Here's how the part is built. I have some questions about the finished solid (model axes, mm). A direction names the side the tool comes from. Round coordinates to 2 decimals unless told otherwise and drop trailing zeros. Loops run counter-clockwise (first coordinate to the right, second up) from the corner with the lowest first, then second, coordinate; pieces in that order, holes last. Notation, with made-up numbers: M 78.5,4.25 L 134.5,4.25 A32 ccw 134.5,39.25 Z; hole C 81.5,1.5 d6. An arc over 180 degrees is marked long. Put each result on its own line as item: value. Start each with the question number.
```python
from build123d import *

# Parameters (mm, degrees)
BOX019_W          = 3
BOX019_H          = 3
BOX019_DEPTH      = 10
CYLINDER022_R     = 3
CYLINDER022_DEPTH = 10
BOX020_W          = 87
BOX020_H          = 45
BOX020_DEPTH      = 12


with BuildPart() as cube019:
    # Box019 → Box019 (new body)
    with BuildSketch(Plane(origin=(-1.5, 2, 0), x_dir=(1, 0, 0), z_dir=(0, 0, 1))):
        with Locations((1.5, 1.5)):
            Rectangle(BOX019_W, BOX019_H)
    extrude(amount=BOX019_DEPTH)


with BuildPart() as fusion010:
    # Cylinder022 → Cylinder022 (new body)
    with BuildSketch(Plane.XY):
        Circle(CYLINDER022_R)
    extrude(amount=CYLINDER022_DEPTH)

    # Fusion010: union Cube019
    add(cube019.part)


with BuildPart() as kegel:
    # Cone → Cone (revolve)
    with BuildSketch(Plane.XZ):
        Polygon((0, 0), (7.5, 0), (10, 10), (0, 10), align=None)
    revolve(axis=Axis((0, 0, 0), (0, 0, 1)))


with BuildPart() as cut006:
    # Cut006 base: copy of Kegel
    add(kegel.part)

    # Cut006: cut Fusion010
    add(fusion010.part, mode=Mode.SUBTRACT)


with BuildPart() as cut006_1:
    # Cut006 placement: moved
    add(cut006.part.moved(Location((0, -21, 0))))


with BuildPart() as cut007:
    # Cut007 base: copy of Kegel
    add(kegel.part)

    # Cut007: cut Fusion010
    add(fusion010.part, mode=Mode.SUBTRACT)


with BuildPart() as cut007_1:
    # Cut007 placement: moved
    add(cut007.part.moved(Location((-42, -21, 0))))


with BuildPart() as cut008:
    # Cut008 base: copy of Kegel
    add(kegel.part)

    # Cut008: cut Fusion010
    add(fusion010.part, mode=Mode.SUBTRACT)


with BuildPart() as cut008_1:
    # Cut008 placement: moved
    add(cut008.part.moved(Location((21, 0, 0))))


with BuildPart() as cut009:
    # Cut009 base: copy of Kegel
    add(kegel.part)

    # Cut009: cut Fusion010
    add(fusion010.part, mode=Mode.SUBTRACT)


with BuildPart() as cut009_1:
    # Cut009 placement: moved
    add(cut009.part.moved(Location((-42, 0, 0))))


with BuildPart() as cut010:
    # Cut010 base: copy of Kegel
    add(kegel.part)

    # Cut010: cut Fusion010
    add(fusion010.part, mode=Mode.SUBTRACT)


with BuildPart() as cut011:
    # Cut011 base: copy of Kegel
    add(kegel.part)

    # Cut011: cut Fusion010
    add(fusion010.part, mode=Mode.SUBTRACT)


with BuildPart() as cut011_1:
    # Cut011 placement: moved
    add(cut011.part.moved(Location((-21, -21, 0))))


with BuildPart() as cut012:
    # Cut012 base: copy of Kegel
    add(kegel.part)

    # Cut012: cut Fusion010
    add(fusion010.part, mode=Mode.SUBTRACT)


with BuildPart() as cut012_1:
    # Cut012 placement: moved
    add(cut012.part.moved(Location((-21, 0, 0))))


with BuildPart() as fusion011:
    # Cut005 base: copy of Kegel
    add(kegel.part)

    # Cut005: cut Fusion010
    add(fusion010.part, mode=Mode.SUBTRACT)


with BuildPart() as fusion011_1:
    # Cut005 placement: moved
    add(fusion011.part.moved(Location((21, -21, 0))))

    # Fusion011: union Cut006, Cut007, Cut008, Cut009, Cut010, Cut011, Cut012
    add(cut006_1.part)
    add(cut007_1.part)
    add(cut008_1.part)
    add(cut009_1.part)
    add(cut010.part)
    add(cut011_1.part)
    add(cut012_1.part)


with BuildPart() as obj1:
    # Box020 → Box020 (new body)
    with BuildSketch(Plane(origin=(-54, -33, -2), x_dir=(1, 0, 0), z_dir=(0, 0, 1))):
        with Locations((43.5, 22.5)):
            Rectangle(BOX020_W, BOX020_H)
    extrude(amount=BOX020_DEPTH)

    # Cut013: cut Fusion011
    add(fusion011_1.part, mode=Mode.SUBTRACT)


solid = obj1.part
```
1) If we mould it in two halves opening along X, with no side actions, what happens to faces 3 (the face through (-42, -20, 10)), 4 (the face through (-48.5, -26, 2.8)), 5 (the face through (-22.5, 4, 5)), 6 (the face through (-54, -11, 4))? For each: pulls with the +X half, pulls with the -X half, needs draft (parallel to the pull), parting line crosses it, or undercut.
2) On a 3-axis mill with a long thin cutter (end or side, diameter ignored), from which of +Z, -Z, +X, -X, +Y, -Y can I reach the whole of each face in a straight line? I mean faces 1 (the face through (21, 1, 10)), 2 (the face through (0, 5, 5)). Say none if no direction works.
3) Suppose I cut it at A-A (z = 1). State how many separate pieces and enclosed holes the cut face has, plus the area to 3 significant figures.
4) Suppose I cut it at B-B (x = 21). Write out the boundary of the cut face in (y, z).
5) If I drill on probe 1 along Y at (x, z) = (-44, 9); probe 2 along Y at (x, z) = (2, 1); probe 3 along X at (y, z) = (-14.5, 8.25), over which ranges is the centre line in solid material (lowest first)? Write a range as from..to.
Results are:
1. face 3: needs draft
1. face 4: undercut
1. face 5: undercut
1. face 6: pulls with the -X half
2. face 1: +Z, +X, -X, +Y, -Y
2. face 2: +Z
3. separate pieces: 9
3. enclosed holes: 8
3. area: 2,680 mm²
4. outline: M -33,-2 L 12,-2 L 12,10 L 10,10 L 7.5,0 L 5,0 L 5,10 L -3,10 L -3,0 L -7.5,0 L -10,10 L -11,10 L -13.5,0 L -16,0 L -16,10 L -24,10 L -24,0 L -28.5,0 L -31,10 L -33,10 Z
5. probe 1: -33..-30.54, -23.24..-18.76, -11.46..-9.54, -2.24..2.24, 9.54..12
5. probe 2: -33..-28.49, -23.24..-18.76, -13.51..-7.49, -2.24..2.24, 7.49..12
5. probe 3: -54..-49.01, -34.99..-28.01, -13.99..-7.01, 7.01..13.99, 28.01..33
